```python
from build123d import *

# Parameters (mm, degrees)
F0_R     = 2.38125
F1_DEPTH = 3.175
F3_DEPTH = 19.05
F5_DEPTH = 25.4
F6_R     = 2.38125
F7_DEPTH = 25.4


with BuildPart() as f1:
    # F0 (on Right) → F1 (new body)
    with BuildSketch(Plane.YZ):
        with BuildLine():
            Line((505.190684, 9.525), (0, 9.525))
            ThreePointArc((0, 9.525), (-9.525, 0), (0, -9.525))
            Line((0, -9.525), (505.190684, -9.525))
            ThreePointArc((505.190684, -9.525), (514.715684, 0), (505.190684, 9.525))
        make_face()
        Circle(F0_R, mode=Mode.SUBTRACT)
        with Locations((252.595342, 0)):
            Circle(F0_R, mode=Mode.SUBTRACT)
        with Locations((505.190684, 0)):
            Circle(F0_R, mode=Mode.SUBTRACT)
    extrude(amount=F1_DEPTH)

    # F2 (on face) → F3 (join)
    with BuildSketch(Plane.XY.offset(9.525)):
        Polygon((-1.5875, 233.545342), (0, 25.4), (0, 479.790684), (-1.5875, 271.645342), align=None)
    extrude(amount=-F3_DEPTH)

    # F4 (on face) → F5 (cut)
    with BuildSketch(Plane.XY.offset(9.525)):
        Polygon((1.5875, 233.557449), (3.175, 25.412107), (3.175, 479.778576), (1.5875, 271.633234), align=None)
    extrude(amount=-F5_DEPTH, mode=Mode.SUBTRACT)

    # F6 (on face) → F7 (cut)
    with BuildSketch(Plane.YZ.offset(1.5875)):
        with Locations((252.595342, 0)):
            Circle(F6_R)
    extrude(amount=-F7_DEPTH, mode=Mode.SUBTRACT)


solid = f1.part
```
Verification items for the finished model (mm, model axes). A direction names the side the tool comes from. Coordinates: 2 decimals unless noted, no trailing zeros. Write each loop counter-clockwise with the first axis right and the second up, starting at its lowest first coordinate (ties: lowest second). Pieces come first, ordered by that corner, then holes. Notation, with made-up numbers: (85.5, -1) - (124.5, -1) arc R19 cw to (124.5, 17) - close; hole circle Ø8 at (63, -5.5). An arc over 180 degrees is marked (long way). Write item = value, one per line.
Q1. Cross-section at A-A (y = 155). Enter the section's corners in (x, z) (3 decimals), plus the area to 3 significant figures.
Answer:
outline = (-0.988, -9.525) - (2.187, -9.525) - (2.187, 9.525) - (-0.988, 9.525) - close
area = 60.5 mm²
Q2. Access from +Z, -Z, +X, -X, +Y, -Y to the whole of each face (thin tool, end or side, straight path). Record for faces 4 (the face through (0, 497, 0)), 5 (the face through (0, 8, 0)), 6 (the face through (1.565, -9.523, 0.209)).
Answer:
face_4 = +Z, -Z, -X, +Y
face_5 = +Z, -Z, -X, -Y
face_6 = +X, -X, -Y
Q3. Material ranges on L1, parallel to X at y = 280, z = -3; L2, parallel to X at y = 24, z = -3 (3 decimals); L3, parallel to Y at x = 0.8, z = -6.5, recorded low to high. Write a range as from..to.
Answer:
L1 = -1.52..1.65
L2 = 0..3.175
L3 = -6.96..512.15
Q4. Go/stop test with flat-tipped pins: pin 1 Ø6 at (y, z) = (338, 3) entering from +X; pin 2 Ø1 at (x, z) = (1.5, 6) entering from -Y; pin 3 Ø1 at (y, z) = (279.5, 7.5) entering from +X. Record where each tip stops, or that it passes through.
Answer:
pin_1 = 2.12
pin_2 = -7.78
pin_3 = 1.65
Q5. Mould release check, pull along Y, two halves, no side actions. Record for faces 1 (the face through (1.588, 249, 0)), 2 (the face through (-1.588, 257, 0)), 3 (the face through (1.565, 514.713, -0.209)): released by +Y, released by -Y, zero draft, split by the parting line, or undercut.
Answer:
face_1 = undercut
face_2 = zero draft
face_3 = released by +Y
